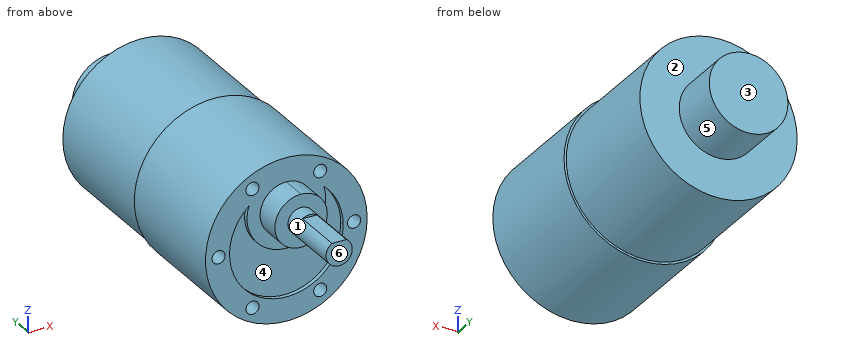
from build123d import *

# Parameters (mm, degrees)
F0_R      = 18.5
F0_R_2    = 18
F0_R_3    = 1.5
F0_R_4    = 3
F1_DEPTH  = 29
F2_R      = 18
F3_DEPTH  = 30
F4_R      = 9
F5_DEPTH  = 12.24
F6_DEPTH  = 6
F7_DEPTH  = 21.5
F8_DEPTH  = 10
F10_DEPTH = 12
F11_DEPTH = 1


with BuildPart() as f1:
    # F0 (on Front) → F1 (new body)
    with BuildSketch(Plane.XZ):
        Circle(F0_R)
        Circle(F0_R_2, mode=Mode.SUBTRACT)
        Circle(F0_R_2)
        with Locations((-7.75, -13.4233937587)):
            Circle(F0_R_3, mode=Mode.SUBTRACT)
        with Locations((7.75, -13.4233937587)):
            Circle(F0_R_3, mode=Mode.SUBTRACT)
        with Locations((-15.5, 0)):
            Circle(F0_R_3, mode=Mode.SUBTRACT)
        with Locations((-7.75, 13.4233937587)):
            Circle(F0_R_3, mode=Mode.SUBTRACT)
        with BuildLine():
            ThreePointArc((-8.5580252347, 9.7857142857), (-4.5708705218, 12.1699278007), (-4.3e-08, 13))
            ThreePointArc((-4.3e-08, 13), (4.5708704815, 12.1699278158), (8.5580252347, 9.7857142857))
            ThreePointArc((8.5580252347, 9.7857142857), (11.8375320074, 5.3733449521), (13, 0))
            ThreePointArc((13, 0), (-5.3733449521, -11.8375320074), (-8.5580252347, 9.7857142857))
        make_face(mode=Mode.SUBTRACT)
        with Locations((15.5, 0)):
            Circle(F0_R_3, mode=Mode.SUBTRACT)
        with Locations((7.75, 13.4233937587)):
            Circle(F0_R_3, mode=Mode.SUBTRACT)
        with BuildLine():
            ThreePointArc((13, 0), (11.8375320074, 5.3733449521), (8.5580252347, 9.7857142857))
            ThreePointArc((8.5580252347, 9.7857142857), (0, -2), (-8.5580252347, 9.7857142857))
            ThreePointArc((-8.5580252347, 9.7857142857), (-5.3733449521, -11.8375320074), (13, 0))
        make_face()
        with BuildLine():
            ThreePointArc((8.5580252347, 9.7857142857), (4.5708704815, 12.1699278158), (-4.3e-08, 13))
            ThreePointArc((-4.3e-08, 13), (-4.5708705218, 12.1699278007), (-8.5580252347, 9.7857142857))
            ThreePointArc((-8.5580252347, 9.7857142857), (0, -2), (8.5580252347, 9.7857142857))
        make_face()
        with BuildLine():
            ThreePointArc((-4.3e-08, 13), (4.2426406719, 11.2426407023), (6, 7))
            ThreePointArc((6, 7), (-4.2426406719, 2.7573592977), (-4.3e-08, 13))
        make_face(mode=Mode.SUBTRACT)
        with BuildLine():
            ThreePointArc((-4.3e-08, 13), (-4.2426406719, 2.7573592977), (6, 7))
            ThreePointArc((6, 7), (4.2426406719, 11.2426407023), (-4.3e-08, 13))
        make_face()
        with Locations((0, 7)):
            Circle(F0_R_4, mode=Mode.SUBTRACT)
        with Locations((0, 7)):
            Circle(F0_R_4)
        with Locations((-15.5, 0)):
            Circle(F0_R_3)
        with Locations((7.75, -13.4233937587)):
            Circle(F0_R_3)
        with Locations((15.5, 0)):
            Circle(F0_R_3)
        with Locations((7.75, 13.4233937587)):
            Circle(F0_R_3)
        with Locations((-7.75, -13.4233937587)):
            Circle(F0_R_3)
        with Locations((-7.75, 13.4233937587)):
            Circle(F0_R_3)
    extrude(amount=-F1_DEPTH)

    # F2 (on face) → F3 (join)
    with BuildSketch(Plane(origin=(0, 29, 0), x_dir=(-1, 0, 0), z_dir=(0, 1, 0))):
        Circle(F2_R)
    extrude(amount=F3_DEPTH)

    # F4 (on face) → F5 (join)
    with BuildSketch(Plane(origin=(0, 59, 0), x_dir=(-1, 0, 0), z_dir=(0, 1, 0))):
        Circle(F4_R)
    extrude(amount=F5_DEPTH)

    # F0 (on Front) → F6 (join)
    with BuildSketch(Plane.XZ):
        with BuildLine():
            ThreePointArc((-4.3e-08, 13), (-4.2426406719, 2.7573592977), (6, 7))
            ThreePointArc((6, 7), (4.2426406719, 11.2426407023), (-4.3e-08, 13))
        make_face()
        with Locations((0, 7)):
            Circle(F0_R_4, mode=Mode.SUBTRACT)
    extrude(amount=F6_DEPTH)

    # F0 (on Front) → F7 (join)
    with BuildSketch(Plane.XZ):
        with Locations((0, 7)):
            Circle(F0_R_4)
    extrude(amount=F7_DEPTH)

    # F0 (on Front) → F8 (cut)
    with BuildSketch(Plane.XZ):
        with Locations((-7.75, 13.4233937587)):
            Circle(F0_R_3)
        with Locations((7.75, 13.4233937587)):
            Circle(F0_R_3)
        with Locations((15.5, 0)):
            Circle(F0_R_3)
        with Locations((-7.75, -13.4233937587)):
            Circle(F0_R_3)
        with Locations((-15.5, 0)):
            Circle(F0_R_3)
        with Locations((7.75, -13.4233937587)):
            Circle(F0_R_3)
    extrude(amount=-F8_DEPTH, mode=Mode.SUBTRACT)

    # F9 (on face) → F10 (cut)
    with BuildSketch(Plane.XZ.offset(21.5)):
        with BuildLine():
            ThreePointArc((-1.6583123952, 9.5), (0, 10), (1.6583123952, 9.5))
            Line((1.6583123952, 9.5), (6.0122050345, 9.5))
            Line((6.0122050345, 9.5), (6.0122050345, 13.4357631467))
            Line((6.0122050345, 13.4357631467), (-7.3503456078, 13.4357631467))
            Line((-7.3503456078, 13.4357631467), (-7.3503456078, 9.5))
            Line((-7.3503456078, 9.5), (-1.6583123952, 9.5))
        make_face()
        with BuildLine():
            Line((-1.6583123952, 9.5), (1.6583123952, 9.5))
            ThreePointArc((1.6583123952, 9.5), (0, 10), (-1.6583123952, 9.5))
        make_face()
    extrude(amount=-F10_DEPTH, mode=Mode.SUBTRACT)

    # F0 (on Front) → F11 (cut)
    with BuildSketch(Plane.XZ):
        with BuildLine():
            ThreePointArc((13, 0), (11.8375320074, 5.3733449521), (8.5580252347, 9.7857142857))
            ThreePointArc((8.5580252347, 9.7857142857), (0, -2), (-8.5580252347, 9.7857142857))
            ThreePointArc((-8.5580252347, 9.7857142857), (-5.3733449521, -11.8375320074), (13, 0))
        make_face()
    extrude(amount=-F11_DEPTH, mode=Mode.SUBTRACT)


solid = f1.part
Design review of the part built by this model. Coordinates are the model's own, in mm. Face numbers are marked on the shaded views. A direction names the side the tool comes from. Round coordinates to 2 decimals unless told otherwise and drop trailing zeros. Write each loop counter-clockwise with the first axis right and the second up, starting at its lowest first coordinate (ties: lowest second). Pieces come first, ordered by that corner, then holes.
Item 1: Wall thickness on L1, parallel to Z at x = -7.75, y = 7.25; L2, parallel to Y at x = 3, z = -2; L3, parallel to Y at x = 15, z = 4: over which ranges is each line inside the solid? List them lowest first.
Item 2: Consider section B-B on y = 55. Give the boundary of the cut face in (x, z).
Item 3: Consider section A-A on z = -6.5. Give the boundary of the cut face in (x, y), and give its area (3 significant figures).
Item 4: Consider section C-C on x = -15.5. Give the boundary of the cut face in (y, z), and give its area (3 significant figures).
Item 5: Draft analysis for pull direction X (two halves, no side actions). For the marked faces 4, 5 and 6, state which applies: released by +X, released by -X, zero draft, split by the parting line, or undercut.
Item 6: For pin 1 Ø1.8 at (x, z) = (-7.75, -13.42) entering from -Y; pin 2 Ø2.5 at (x, z) = (-15.5, 0.5) entering from -Y; pin 3 Ø1.8 at (x, z) = (-7.75, 13.42) entering from +Y; pin 4 Ø12 at (y, z) = (10, -2.5) entering from +X, all flat-tipped, find the tip position at first contact; note any pin that passes through.
Item 7: Consider section D-D on y = 26.5. Give the boundary of the cut face in (x, z), and give its area (3 significant figures).
Item 8: For the marked faces 1, 2 and 3, list the 3-axis set-ups (+Z, -Z, +X, -X, +Y, -Y) from which the entire face can be reached by the end or side of a thin tool; tool diameter is ignored.
Check values:
1. L1: z = -16.8 to -14.92, -11.92 to 11.92, 14.92 to 16.8
1. L2: y = 1 to 71.24
1. L3: y = 0 to 59
2. outline: circle Ø36 at (0, 0)
3. outline: (-17.32, 0) - (-11.26, 0) - (-11.26, 1) - (11.26, 1) - (11.26, 0) - (17.32, 0) - (17.32, 29) - (16.79, 29) - (16.79, 59) - (6.22, 59) - (6.22, 71.24) - (-6.22, 71.24) - (-6.22, 59) - (-16.79, 59) - (-16.79, 29) - (-17.32, 29) - close
3. area: 2,140 mm2
4. outline: (0, -10.1) - (29, -10.1) - (29, -9.15) - (59, -9.15) - (59, 9.15) - (29, 9.15) - (29, 10.1) - (0, 10.1) - (0, 1.5) - (10, 1.5) - (10, -1.5) - (0, -1.5) - close
4. area: 1,100 mm2
5. face 4: undercut
5. face 5: split by the parting line
5. face 6: zero draft
6. pin 1: stops at y = 10
6. pin 2: stops at y = 0
6. pin 3: stops at y = 59
6. pin 4: stops at x = 18.5
7. outline: circle Ø37 at (0, 0)
7. area: 1,080 mm2
8. face 1: -Y
8. face 2: +Y
8. face 3: +Z, -Z, +X, -X, +Y
